Design review of the part built by this model. Coordinates are the model's own, in mm. A direction names the side the tool comes from. Coordinates: 2 decimals unless noted, no trailing zeros. Loops run counter-clockwise (first coordinate to the right, second up) from the corner with the lowest first, then second, coordinate; pieces in that order, holes last. Notation, with made-up numbers: M -39,67 L -3,67 A18 ccw -3,84 Z; hole C 68.5,25.25 d6. An arc over 180 degrees is marked long. Write item = value, one per line. Start each with the question number.
from build123d import *

# Parameters (mm, degrees)
BOSS_EXTRUDE1_DEPTH = 4
SKETCH2_W           = 5
SKETCH2_H           = 10
BOSS_EXTRUDE2_DEPTH = 15
BOSS_EXTRUDE3_REACH = 137.403
SKETCH3_W           = 5
SKETCH3_H           = 5
FILLET1_R           = 2


with BuildPart() as part:
    # Sketch1 → Boss-Extrude1 (new body)
    with BuildSketch(Plane(origin=(0, 0, 0), x_dir=(1, 0, 0), z_dir=(0, 1, 0))):
        with BuildLine():
            Line((0, 87), (0, 40))
            ThreePointArc((0, 40), (-40, 0), (0, -40))
            Line((0, -40), (0, -87))
            ThreePointArc((0, -87), (-87, 0), (0, 87))
        make_face()
    extrude(amount=BOSS_EXTRUDE1_DEPTH)

    # Sketch2 → Boss-Extrude2 (add)
    with BuildSketch(Plane(origin=(0, 4, 0), x_dir=(1, 0, 0), z_dir=(0, 1, 0))):
        with Locations((-74.5, -20)):
            Rectangle(SKETCH2_W, SKETCH2_H)
        with Locations((-74.5, 20)):
            Rectangle(SKETCH2_W, SKETCH2_H)
    extrude(amount=BOSS_EXTRUDE2_DEPTH)

    # Sketch3 → Boss-Extrude3 (add, up to next)
    with BuildSketch(Plane.XY.offset(-15), mode=Mode.PRIVATE) as boss_extrude3_sk1:
        with Locations((-74.5, 16.5)):
            Rectangle(SKETCH3_W, SKETCH3_H)
    boss_extrude3_tool1 = extrude(boss_extrude3_sk1.sketch, amount=BOSS_EXTRUDE3_REACH, mode=Mode.PRIVATE) - part.part
    add(boss_extrude3_tool1.solids().sort_by_distance((-74.5, 16.5, -15))[0])

    # Fillet1
    fillet1_edges = [part.edges().sort_by_distance(p)[0] for p in [
        (-77, 11.5, 25),
        (-72, 11.5, 25),
        (-77, 19, 0),
        (-74.5, 19, 25),
        (-72, 19, 0),
        (-77, 11.5, -25),
        (-72, 11.5, -25),
        (-74.5, 19, -25),
        (-72, 9, -15),
        (-77, 9, -15),
        (-77, 9, 15),
        (-72, 9, 15),
        (-72, 14, 0),
        (-77, 14, 0),
        (-74.5, 14, -15),
    ]]
    fillet(fillet1_edges, radius=FILLET1_R)


solid = part.part
Q1. Mouldability with a two-part tool opening along Z and no side actions: class faces 4 (the face through (-43, 0, -1)), 5 (the face through (-39.99, 1.97, -0.88)), 6 (the face through (-86.98, 1.97, 1.91)) as released by +Z, released by -Z, zero draft, split by the parting line, or undercut.
Q2. For faces 1 (the face through (0, 2, 63)), 2 (the face through (-77, 16.2, -1.8)), 3 (the face through (-72, 16.2, -1.8)), list the 3-axis set-ups (+Z, -Z, +X, -X, +Y, -Y) from which the entire face can be reached by the end or side of a thin tool; tool diameter is ignored.
Q3. Add section B-B on y = 6.75. State the section outline as (x, z) points, plus the area to 3 significant figures.
Q4. Add section D-D on x = -60.5. State the section outline as (y, z) points, plus the area to 3 significant figures.
Q5. To check wall thickness, follow line 1 (Z direction, x = -75, y = 6); line 2 (Y direction, x = -54, z = -48.5); line 3 (Z direction, x = -23.5, y = 1.25). State the ranges of each line that lie inside material, in increasing order. Write a range as from..to.
Q6. Clearance check with flat-ended pins moving along their axes: P1, Ø10.5, axis at y = 13, z = -5, coming from the +X side; P2, Ø4, axis at x = -42, z = 3, coming from the +Y side; P3, Ø2, axis at x = -69.5, y = 5.5, coming from the -Z side; P4, Ø1.1, axis at x = -74.5, y = 8, coming from the +Z side. State where each tip first meets the part, or that it passes through.
Q7. Add section C-C on x = -25.5. State the section outline as (y, z) points, plus the area to 3 significant figures.
Q8. Add section A-A on z = 0. State the section outline as (x, y) points, plus the area to 3 significant figures.
Values follow:
q1.face_4 = zero draft
q1.face_5 = undercut
q1.face_6 = split by the parting line
q2.face_1 = +Z, -Z, +X, +Y, -Y
q2.face_2 = +Z, -Z, -X, +Y
q2.face_3 = +Z, -Z, +X, +Y
q3.outline = M -77,-23 A2 ccw -75,-25 L -74,-25 A2 ccw -72,-23 L -72,-17 A2 ccw -74,-15 L -75,-15 A2 ccw -77,-17 Z; M -77,17 A2 ccw -75,15 L -74,15 A2 ccw -72,17 L -72,23 A2 ccw -74,25 L -75,25 A2 ccw -77,23 Z
q3.area = 93.1 mm2
q4.outline = M 0,-62.52 L 4,-62.52 L 4,62.52 L 0,62.52 Z
q4.area = 500 mm2
q5.line_1 = -25..-15, 15..25
q5.line_2 = 0..4
q5.line_3 = -83.77..-32.37, 32.37..83.77
q6.P1 = -72
q6.P2 = 4
q6.P3 = through
q6.P4 = 25
q7.outline = M 0,-83.18 L 4,-83.18 L 4,-30.82 L 0,-30.82 Z; M 0,30.82 L 4,30.82 L 4,83.18 L 0,83.18 Z
q7.area = 419 mm2
q8.outline = M -87,0 L -40,0 L -40,4 L -87,4 Z; M -77,16 A2 ccw -75,14 L -74,14 A2 ccw -72,16 L -72,17 A2 ccw -74,19 L -75,19 A2 ccw -77,17 Z
q8.area = 210 mm2
